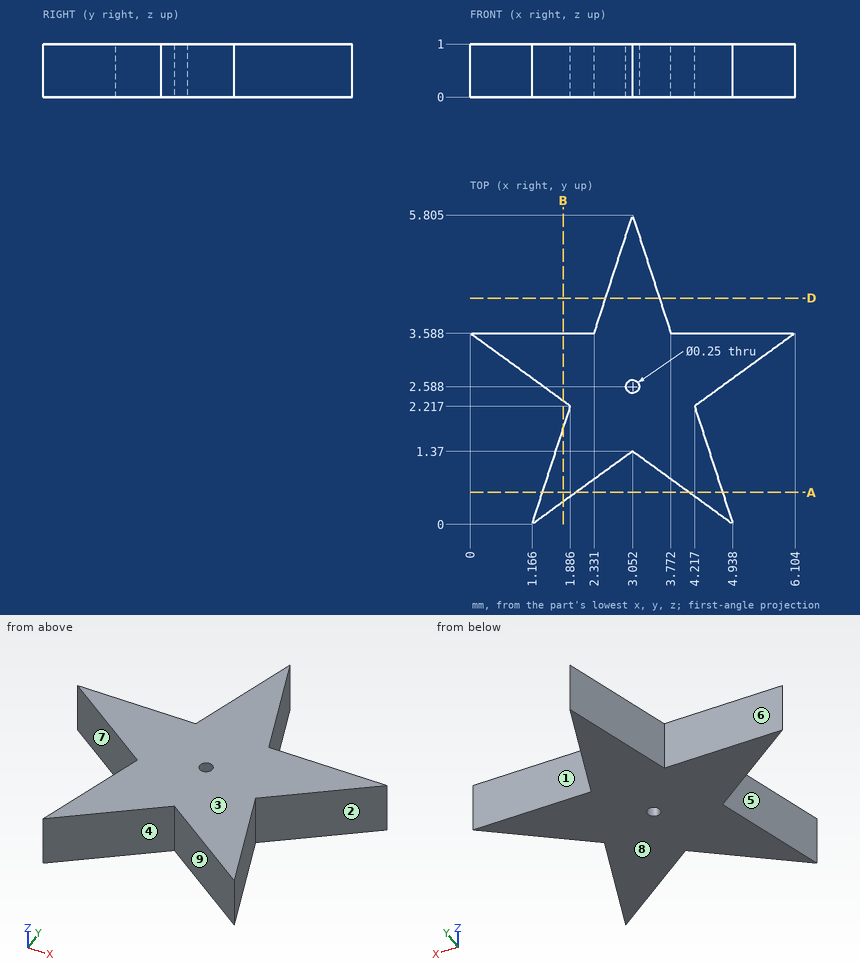
Print and shaded views of the part. All mm, measured from the part's lowest x, y and z. A direction names the side the tool comes from. Round coordinates to 2 decimals unless told otherwise and drop trailing zeros. Write each loop counter-clockwise with the first axis right and the second up, starting at its lowest first coordinate (ties: lowest second). Pieces come first, ordered by that corner, then holes. Notation, with made-up numbers: (51.5, 3) -> (98.5, 3) arc R22 cw to (98.5, 39) -> close; hole circle Ø4 at (-24, 37.5). An arc over 180 degrees is marked (long way). Return JSON: item names as keys, results as strings. Group by question number.
Q1. Pin check, flat tips, straight feed: pin 1 (2 mm diameter, centred on x = 1.5, y = 2.5, fed in from -Z); pin 2 (0.5 mm diameter, centred on x = 4.5, z = 0.5, fed in from +Y). Stop position of each tip, or through.
Q2. Probe L1, parallel to X at y = 1.1, z = 0.7 (1 decimal); L2, parallel to X at y = 0.7, z = 0.7 (1 decimal); L3, parallel to Y at x = 5, z = 0.55 (1 decimal). List the from-to ranges inside material, lowest first. Write a range as [from, to].
Q3. Which spindle directions (+Z, -Z, +X, -X, +Y, -Y) get a long thin tool onto all of the face, cutting with end or side? Do the marked faces 1, 2, 3, 4 and 5. Say none if no direction does.
Q4. Mould opens along Y. For the marked faces 6, 7, 8 and 9 say: pulls with the +Y half, pulls with the -Y half, needs draft (parallel to the pull), parting line crosses it, or undercut.
Q5. Saw through at D-D on y = 4.25. Write the cut outline in (x, z), plus the area to 3 significant figures.
Q6. Saw through at A-A on y = 0.6. Write the cut outline in (x, z).
Q7. Saw through at B-B on x = 1.75. Write the cut outline in (y, z) (1 decimal).
Answer:
{
 "1": {"pin 1": "z = 0", "pin 2": "y = 3.59"},
 "2": {"L1": "[1.5, 2.7], [3.4, 4.6]", "L2": "[1.4, 2.1], [4, 4.7]", "L3": "[2.8, 3.6]"},
 "3": {"face 1": "+Z, -Z, +X, +Y", "face 2": "+Z, -Z, +X", "face 3": "+Z, +X, -X, +Y, -Y", "face 4": "+Z, -Z, -Y", "face 5": "+Z, -Z, -X"},
 "4": {"face 6": "pulls with the +Y half", "face 7": "undercut", "face 8": "needs draft", "face 9": "pulls with the -Y half"},
 "5": {"outline": "(2.55, 0) -> (3.56, 0) -> (3.56, 1) -> (2.55, 1) -> close", "area": "1.01 mm2"},
 "6": {"outline": "(1.36, 0) -> (1.99, 0) -> (1.99, 1) -> (1.36, 1) -> close; (4.11, 0) -> (4.74, 0) -> (4.74, 1) -> (4.11, 1) -> close"},
 "7": {"outline": "(0.4, 0) -> (1.8, 0) -> (1.8, 1) -> (0.4, 1) -> close; (2.3, 0) -> (3.6, 0) -> (3.6, 1) -> (2.3, 1) -> close"}
}
